from build123d import *

# Parameters (mm, degrees)
CROQUIS1_R              = 0.5
SALIENTE_EXTRUIR1_DEPTH = 1.5
CROQUIS2_R              = 3.5
CROQUIS2_R_2            = 2.25
SALIENTE_EXTRUIR2_DEPTH = 2.5
CROQUIS3_R              = 2.5
CORTAR_EXTRUIR1_DEPTH   = 1
CROQUIS4_R              = 1
CORTAR_EXTRUIR2_DEPTH   = 1


with BuildPart() as part:
    # Croquis1 → Saliente-Extruir1 (new body)
    with BuildSketch(Plane(origin=(0, 0, 0), x_dir=(1, 0, 0), z_dir=(0, 1, 0))):
        with BuildLine():
            Line((-3.5, 0), (-2, -14.5))
            ThreePointArc((-2, -14.5), (0, -16.5), (2, -14.5))
            Line((2, -14.5), (3.5, 0))
            ThreePointArc((3.5, 0), (0, 3.5), (-3.5, 0))
        make_face()
        with Locations(Location((0, -14.5, 0), (0, 0, 270))):
            Circle(CROQUIS1_R, mode=Mode.SUBTRACT)
        with Locations(Location((0, -12.5, 0), (0, 0, 270))):
            Circle(CROQUIS1_R, mode=Mode.SUBTRACT)
        with Locations(Location((0, -10.5, 0), (0, 0, 270))):
            Circle(CROQUIS1_R, mode=Mode.SUBTRACT)
        with Locations(Location((0, -8.5, 0), (0, 0, 270))):
            Circle(CROQUIS1_R, mode=Mode.SUBTRACT)
        with Locations(Location((0, -6.5, 0), (0, 0, 270))):
            Circle(CROQUIS1_R, mode=Mode.SUBTRACT)
        with Locations(Location((0, -4.5, 0), (0, 0, 270))):
            Circle(CROQUIS1_R, mode=Mode.SUBTRACT)
    extrude(amount=SALIENTE_EXTRUIR1_DEPTH)

    # Croquis2 → Saliente-Extruir2 (add)
    with BuildSketch(Plane(origin=(0, 1.5, 0), x_dir=(1, 0, 0), z_dir=(0, 1, 0))):
        with Locations(Location((0, 0, 0), (0, 0, 180))):
            Circle(CROQUIS2_R)
        with Locations(Location((0, 0, 0), (0, 0, 270))):
            Circle(CROQUIS2_R_2, mode=Mode.SUBTRACT)
    extrude(amount=SALIENTE_EXTRUIR2_DEPTH)

    # Croquis3 → Cortar-Extruir1 (cut)
    with BuildSketch(Plane.XZ):
        with Locations(Location((0, 0, 0), (0, 0, 270))):
            Circle(CROQUIS3_R)
    extrude(amount=-CORTAR_EXTRUIR1_DEPTH, mode=Mode.SUBTRACT)

    # Croquis4 → Cortar-Extruir2 (cut)
    with BuildSketch(Plane(origin=(0, 1.5, 0), x_dir=(1, 0, 0), z_dir=(0, 1, 0))):
        with Locations(Location((0, 0, 0), (0, 0, 270))):
            Circle(CROQUIS4_R)
    extrude(amount=-CORTAR_EXTRUIR2_DEPTH, mode=Mode.SUBTRACT)


solid = part.part
Read the model definition and answer for the solid it produces. Units are mm, in the model's axes. A direction names the side the tool comes from. Coordinates: 2 decimals unless noted, no trailing zeros. Order: outer loops, then holes, each group sorted by start corner. A loop starts at its lowest first (then second) coordinate and runs counter-clockwise, first axis right, second up. Notation, with made-up numbers: (66.25, 78.5) -> (119.25, 78.5) arc R16 ccw to (119.25, 101.5) -> close; hole circle Ø3 at (-20, -39.5). An arc over 180 degrees is marked (long way). Answer as a JSON object with one key per item and string values.
1) A cutting plane is placed at A-A, the plane z = 4.5. Determine the outline of the cut face in (x, y).
Model answer:
{"outline": "(-3.03, 0) -> (-0.5, 0) -> (-0.5, 1.5) -> (-3.03, 1.5) -> close; (0.5, 0) -> (3.03, 0) -> (3.03, 1.5) -> (0.5, 1.5) -> close"}
2) A cutting plane is placed at C-C, the plane z = 10.5. Determine the outline of the cut face in (x, y), plus the area to 3 significant figures.
Model answer:
{"outline": "(-2.41, 0) -> (-0.5, 0) -> (-0.5, 1.5) -> (-2.41, 1.5) -> close; (0.5, 0) -> (2.41, 0) -> (2.41, 1.5) -> (0.5, 1.5) -> close", "area": "5.74 mm²"}
3) A cutting plane is placed at B-B, the plane y = 3.2. Determine the outline of the cut face in (x, z), plus the area to 3 significant figures.
Model answer:
{"outline": "circle Ø7 at (0, 0); hole circle Ø4.5 at (0, 0)", "area": "22.6 mm²"}
4) Each of these flat-tipped pins is pushed along its axis until it touches: pin 1 (3 mm diameter, centred on x = 0, z = 0, fed in from -Y); pin 2 (1 mm diameter, centred on y = 1, z = 5.5, fed in from -X); pin 3 (1 mm diameter, centred on x = -0.5, z = -1.5, fed in from +Y). Where does it stop, or does it pass through?
Model answer:
{"pin 1": "stops at y = 1", "pin 2": "stops at x = -2.98", "pin 3": "stops at y = 1.5"}
5) Consider line 1 along X through (y, z) = (2.55, 0); line 2 along X through (y, z) = (0.5, 0); line 3 along Z through (x, y) = (-0.5, 3.5). Determine where each line is inside the solid, lowest interval first. Write a range as from..to.
Model answer:
{"line 1": "x = -3.5..-2.25, 2.25..3.5", "line 2": "x = -3.5..-2.5, 2.5..3.5", "line 3": "z = -3.46..-2.19, 2.19..3.46"}
6) The mould has two halves that part along X. Classify faces 4 (the face through (0, 1, 9)), 5 (the face through (-2.76, 0.74, 7.15)), 6 (the face through (1, 1.5, 8)): released by +X, released by -X, zero draft, split by the parting line, or undercut.
Model answer:
{"face 4": "undercut", "face 5": "released by -X", "face 6": "zero draft"}
7) A tool of negligible diameter and unlimited length cuts with its end or side. For faces 1 (the face through (-1, 1, -1)), 2 (the face through (0, 1, 15)), 3 (the face through (0.676, 2.732, 2.146)), from which of +Z, -Z, +X, -X, +Y, -Y can it reach the whole face along a straight path? Write none if from no direction.
Model answer:
{"face 1": "-Y", "face 2": "+Y, -Y", "face 3": "+Y"}
